Part model, mm, in its own coordinate system. Face numbers are marked on the shaded views. A direction names the side the tool comes from. Give positions to 0.01 mm unless a question says otherwise; leave off trailing zeros. Write each loop counter-clockwise with the first axis right and the second up, starting at its lowest first coordinate (ties: lowest second). Pieces come first, ordered by that corner, then holes. Notation, with made-up numbers: (76, -13) - (103, -13) arc R24 cw to (103, 17) - close; hole circle Ø10 at (48.25, 88.5). An arc over 180 degrees is marked (long way). Answer as a JSON object with one key per item and string values. Group by question number.
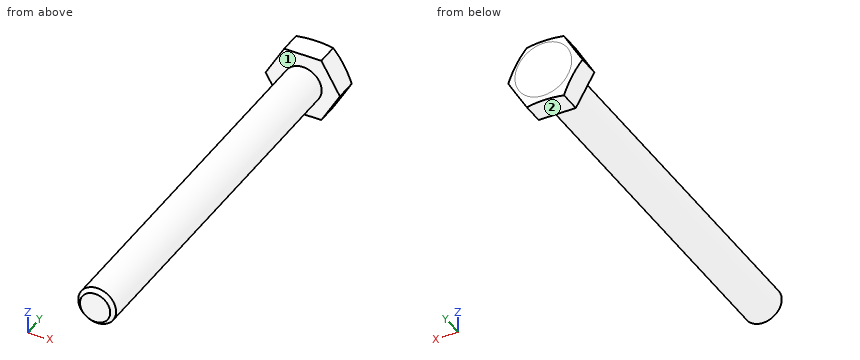
```python
from build123d import *

# Parameters (mm, degrees)
EXTRUDE_1_DEPTH = 6.7
SKETCH_4_R      = 5
EXTRUDE_2_DEPTH = 100
CHAMFER_1_SIZE  = 1


with BuildPart() as part:
    # 草图2 → 凸台-拉伸1 (new body)
    with BuildSketch(Plane(origin=(0, 0, 0), x_dir=(1, 0, 0), z_dir=(0, 1, 0))):
        Polygon((9.814954576, 0), (4.907477288, 8.5), (-4.907477288, 8.5), (-9.814954576, 0), (-4.907477288, -8.5), (4.907477288, -8.5), align=None)
    extrude(amount=EXTRUDE_1_DEPTH)

    # 草图3 → 切除-旋转1 (revolve, cut)
    with BuildSketch(Plane.XY, mode=Mode.PRIVATE) as cut_revolve_1_sk:
        Polygon((-9.814954576, 5.7), (-7.5, 6.7), (-9.814954576, 6.7), align=None)
    revolve(cut_revolve_1_sk.sketch.rotate(Axis((0, 0, 0), (0, 1, 0)), 270), axis=Axis((0, 0, 0), (0, 1, 0)), mode=Mode.SUBTRACT)

    # 草图4 → 凸台-拉伸2 (add)
    with BuildSketch(Plane.XZ):
        with Locations(Location((0, 0, 0), (0, 0, 270))):
            Circle(SKETCH_4_R)
    extrude(amount=EXTRUDE_2_DEPTH)

    # 倒角1
    chamfer_1_edges = [part.edges().sort_by_distance(p)[0] for p in [
        (0, -100, 5),
    ]]
    chamfer(chamfer_1_edges, length=CHAMFER_1_SIZE)


solid = part.part
```
1) Probe line 1 (Y direction, x = 0.5, z = -6.25); line 2 (X direction, y = -73, z = 3); line 3 (Z direction, x = 1, y = -33.5). List the from-to ranges inside material, lowest first.
2) Drop flat-ended pins along their axis: P1, Ø3, axis at x = -5, y = -46, coming from the +Z side; P2, Ø2, axis at x = -0.5, y = -53, coming from the +Z side; P3, Ø2, axis at x = 4, y = -11.5, coming from the +Z side. Give the stop position or say it passes through.
3) Which spindle directions (+Z, -Z, +X, -X, +Y, -Y) get a long thin tool onto all of the face, cutting with end or side? Do the marked faces 1 and 2. Say none if no direction does.
4) Band-saw the part on B-B (y = -12). List the corners of the cut face in (x, z).
5) Band-saw the part on A-A (x = 0). List the corners of the cut face in (y, z).
Verdict:
{
 "1": {"line 1": "0 to 6.7", "line 2": "-4 to 4", "line 3": "-4.9 to 4.9"},
 "2": {"P1": "z = 3.57", "P2": "z = 5", "P3": "z = 4"},
 "3": {"face 1": "-Y", "face 2": "-Z, +X, -X, +Y, -Y"},
 "4": {"outline": "circle Ø10 at (0, 0)"},
 "5": {"outline": "(-100, -4) - (-99, -5) - (0, -5) - (0, -8.5) - (6.27, -8.5) - (6.7, -7.5) - (6.7, 7.5) - (6.27, 8.5) - (0, 8.5) - (0, 5) - (-99, 5) - (-100, 4) - close"}
}
